Build history of the part. All positions in model axes, mm. A direction names the side the tool comes from. Coordinates: 2 decimals unless noted, no trailing zeros. Loops run counter-clockwise (first coordinate to the right, second up) from the corner with the lowest first, then second, coordinate; pieces in that order, holes last.
(1) Slice it at B-B (x = 0). Give the cut face in (y, z), and give its area (3 significant figures).
(2) Slice it at C-C (z = 104). Give the cut face in (x, y), and give its area (3 significant figures).
(3) Slice it at D-D (y = 9.5). Give the cut face in (x, z), and give its area (3 significant figures).
(4) Wall check: L1, parallel to X at y = -1, z = 56.5; L2, parallel to X at y = -3, z = 101; L3, parallel to Y at x = -10.5, z = 156.5. Give the ranges that are in metal, low to high.
(5) Slice it at A-A (y = 0). Give the cut face in (x, z), and give its area (3 significant figures).
(6) Flat gauge pins, fed straight in: P1, Ø4.5, axis at y = 15.5, z = 218, coming from the +X side; P2, Ø3.5, axis at y = 13.5, z = 214, coming from the -X side; P3, Ø2, axis at x = -3, z = 86.5, coming from the -Y side; P4, Ø3.5, axis at x = -1, y = 14, coming from the -Z side. Where does each tip first touch, or does it go through?
(7) Two-plate mould, pull along Z, no slides. Class faces 5 (the face through (0, 15, 199.39)), 6 (the face through (0, 16.51, 221)), 7 (the face through (6.14, -11.32, 12.7)): pulls with the +Z half, pulls with the -Z half, needs draft (parallel to the pull), parting line crosses it, or undercut.
(8) Tool access for faces 1 (the face through (2.54, 15, 221)), 2 (the face through (-2.75, -12.4, 6.26)), 3 (the face through (-2.54, 14, 221)), 4 (the face through (0, -1, 243.84)): list every direction of +Z, -Z, +X, -X, +Y, -Y with a clear straight run to the whole face (end or side of a thin tool).
from build123d import *

# Parameters (mm, degrees)
SKETCH1_R           = 12.7
BOSS_EXTRUDE1_DEPTH = 12.7
SKETCH2_R           = 13.97
BOSS_EXTRUDE2_DEPTH = 2.54
SKETCH3_R           = 12.7
BOSS_EXTRUDE3_DEPTH = 228.6
BOSS_EXTRUDE4_START = -44.45
BOSS_EXTRUDE4_DEPTH = 44.45


with BuildPart() as part:
    # Sketch1 → Boss-Extrude1 (new body)
    with BuildSketch(Plane.XY):
        Circle(SKETCH1_R)
    extrude(amount=BOSS_EXTRUDE1_DEPTH)

    # Sketch2 → Boss-Extrude2 (add)
    with BuildSketch(Plane.XY.offset(12.7)):
        Circle(SKETCH2_R)
    extrude(amount=BOSS_EXTRUDE2_DEPTH)

    # Sketch3 → Boss-Extrude3 (add)
    with BuildSketch(Plane.XY.offset(15.24)):
        Circle(SKETCH3_R)
    extrude(amount=BOSS_EXTRUDE3_DEPTH)

    # Sketch4 → Boss-Extrude4 (add)
    with BuildSketch(Plane.XY.offset(243.84).offset(BOSS_EXTRUDE4_START)):
        with BuildLine():
            Line((-2.54, 16.51), (2.54, 16.51))
            Line((2.54, 16.51), (2.54, 12.443407893))
            ThreePointArc((2.54, 12.443407893), (0, 12.7), (-2.54, 12.443407893))
            Line((-2.54, 12.443407893), (-2.54, 16.51))
        make_face()
    extrude(amount=BOSS_EXTRUDE4_DEPTH)


solid = part.part
Response values:
1. outline: (-13.97, 12.7) - (-12.7, 12.7) - (-12.7, 0) - (12.7, 0) - (12.7, 12.7) - (13.97, 12.7) - (13.97, 15.24) - (12.7, 15.24) - (12.7, 199.39) - (16.51, 199.39) - (16.51, 243.84) - (-12.7, 243.84) - (-12.7, 15.24) - (-13.97, 15.24) - close
1. area: 6,370 mm2
2. outline: circle Ø25.4 at (0, 0)
2. area: 507 mm2
3. outline: (-10.24, 12.7) - (-8.43, 12.7) - (-8.43, 0) - (8.43, 0) - (8.43, 12.7) - (10.24, 12.7) - (10.24, 15.24) - (8.43, 15.24) - (8.43, 243.84) - (-8.43, 243.84) - (-8.43, 15.24) - (-10.24, 15.24) - close
3. area: 4,120 mm2
4. L1: x = -12.66 to 12.66
4. L2: x = -12.34 to 12.34
4. L3: y = -7.14 to 7.14
5. outline: (-13.97, 12.7) - (-12.7, 12.7) - (-12.7, 0) - (12.7, 0) - (12.7, 12.7) - (13.97, 12.7) - (13.97, 15.24) - (12.7, 15.24) - (12.7, 243.84) - (-12.7, 243.84) - (-12.7, 15.24) - (-13.97, 15.24) - close
5. area: 6,200 mm2
6. P1: stops at x = 2.54
6. P2: stops at x = -4.82
6. P3: stops at y = -12.54
6. P4: stops at z = 0
7. face 5: undercut
7. face 6: needs draft
7. face 7: pulls with the -Z half
8. face 1: +Z, +X, +Y
8. face 2: -Z
8. face 3: +Z, -X, +Y
8. face 4: +Z, +X, -X, +Y, -Y
